Geometry check sheet. Reference: the model listing, model coordinates, mm. A direction names the side the tool comes from. Coordinates: 2 decimals unless noted, no trailing zeros. Loops run counter-clockwise (first coordinate to the right, second up) from the corner with the lowest first, then second, coordinate; pieces in that order, holes last.
from build123d import *

# Parameters (mm, degrees)
X_Z_SEVO_MOUNT_SKETCH_R            = 12.7
X_Z_SERVO_MOUNT_DEPTH              = 3.175
BASE_MOUNT_SKETCH_W                = 3.175
BASE_MOUNT_SKETCH_H                = 4.233333334
BASE_MOUNT_DEPTH                   = 4.175
SERVO_HORN_MOUNTING_HOLES_SKETCH_R = 0.3175
SERVO_HORN_MOUNT_HOLES_DEPTH       = 4.175


with BuildPart() as part:
    # X-Z Sevo Mount Sketch → X-Z Servo Mount (new body)
    with BuildSketch(Plane(origin=(0, 0, 0), x_dir=(1, 0, 0), z_dir=(0, 1, 0))):
        Circle(X_Z_SEVO_MOUNT_SKETCH_R)
    extrude(amount=X_Z_SERVO_MOUNT_DEPTH)

    # Base Mount Sketch → Base Mount (cut, through all)
    with BuildSketch(Plane(origin=(0, 3.175, 0), x_dir=(1, 0, 0), z_dir=(0, 1, 0))):
        Rectangle(BASE_MOUNT_SKETCH_W, BASE_MOUNT_SKETCH_H)
    extrude(amount=-BASE_MOUNT_DEPTH, mode=Mode.SUBTRACT)

    # Servo Horn Mounting Holes Sketch → Servo Horn Mount Holes (cut, through all)
    with BuildSketch(Plane.XZ):
        with Locations((0, 8.1661)):
            Circle(SERVO_HORN_MOUNTING_HOLES_SKETCH_R)
        with Locations((2.794, 8.1661)):
            Circle(SERVO_HORN_MOUNTING_HOLES_SKETCH_R)
        with Locations((-2.794, 8.1661)):
            Circle(SERVO_HORN_MOUNTING_HOLES_SKETCH_R)
        with Locations((2.794, -8.1661)):
            Circle(SERVO_HORN_MOUNTING_HOLES_SKETCH_R)
        with Locations((0, -8.1661)):
            Circle(SERVO_HORN_MOUNTING_HOLES_SKETCH_R)
        with Locations((-2.794, -8.1661)):
            Circle(SERVO_HORN_MOUNTING_HOLES_SKETCH_R)
        with Locations((8.1661, 0)):
            Circle(SERVO_HORN_MOUNTING_HOLES_SKETCH_R)
        with Locations((8.1661, 2.794)):
            Circle(SERVO_HORN_MOUNTING_HOLES_SKETCH_R)
        with Locations((8.1661, -2.794)):
            Circle(SERVO_HORN_MOUNTING_HOLES_SKETCH_R)
        with Locations((-8.1661, -2.794)):
            Circle(SERVO_HORN_MOUNTING_HOLES_SKETCH_R)
        with Locations((-8.1661, 2.794)):
            Circle(SERVO_HORN_MOUNTING_HOLES_SKETCH_R)
        with Locations((-8.1661, 0)):
            Circle(SERVO_HORN_MOUNTING_HOLES_SKETCH_R)
    extrude(amount=-SERVO_HORN_MOUNT_HOLES_DEPTH, mode=Mode.SUBTRACT)


solid = part.part
(1) Scan lines: L1, parallel to Z at x = 0, y = 1.05; L2, parallel to X at y = 1.45, z = -3; L3, parallel to X at y = 2.95, z = -0.5. Record each from-to range of solid material in increasing order.
Findings:
L1: z = -12.7 to -8.48, -7.85 to -2.12, 2.12 to 7.85, 8.48 to 12.7
L2: x = -12.34 to -8.41, -7.92 to 7.92, 8.41 to 12.34
L3: x = -12.69 to -1.59, 1.59 to 12.69
(2) Gauge pin test, flat end, axial feed: pin 1 Ø1 at (x, y) = (-1.5, 1) entering from +Z. Record the tip position at first contact, or that the pin passes through.
Findings:
pin 1: stops at z = 12.66
(3) Sectioned sample at B-B on z = 0. Record the cut outline in (x, y) (1 decimal).
Findings:
outline: (-12.7, 0) - (-8.5, 0) - (-8.5, 3.2) - (-12.7, 3.2) - close; (-7.8, 0) - (-1.6, 0) - (-1.6, 3.2) - (-7.8, 3.2) - close; (1.6, 0) - (7.8, 0) - (7.8, 3.2) - (1.6, 3.2) - close; (8.5, 0) - (12.7, 0) - (12.7, 3.2) - (8.5, 3.2) - close
(4) Access from +Z, -Z, +X, -X, +Y, -Y to the whole of each face (thin tool, end or side, straight path). Record for faces 1 (the flat face through (0, 0, -3)), 2 (the flat face through (0, 2, -2.117)).
Findings:
face 1: +Z, -Z, +X, -X, -Y
face 2: +Y, -Y
(5) Sectioned sample at D-D on z = -7.25. Record the cut outline in (x, y) (3 decimals), and give its area (3 significant figures).
Findings:
outline: (-10.427, 0) - (10.427, 0) - (10.427, 3.175) - (-10.427, 3.175) - close
area: 66.2 mm2
(6) Draft check along X on faces 3 (the flat face through (0, 2, 2.117)), 4 (the cylindrical face through (-2.75, 1.57, 12.4)), 5 (the flat face through (0, 3.175, -3)). Enter one of: +X half, -X half, draft (parallel to the pull), parting line (faces both ways), or undercut.
Findings:
face 3: undercut
face 4: parting line
face 5: draft
(7) Sectioned sample at C-C on y = 1.45. State how many separate pieces and enclosed holes the cut face has, and give its area (3 significant figures).
Findings:
separate pieces: 1
enclosed holes: 13
area: 489 mm2
(8) Sectioned sample at A-A on x = 0. Record the cut outline in (y, z) (3 decimals), and give its area (3 significant figures).
Findings:
outline: (0, -12.7) - (3.175, -12.7) - (3.175, -8.484) - (0, -8.484) - close; (0, -7.849) - (3.175, -7.849) - (3.175, -2.117) - (0, -2.117) - close; (0, 2.117) - (3.175, 2.117) - (3.175, 7.849) - (0, 7.849) - close; (0, 8.484) - (3.175, 8.484) - (3.175, 12.7) - (0, 12.7) - close
area: 63.2 mm2
